Geometry check sheet. Reference: the model listing, model coordinates, mm. Coordinates: 2 decimals unless noted, no trailing zeros. Write each loop counter-clockwise with the first axis right and the second up, starting at its lowest first coordinate (ties: lowest second). Pieces come first, ordered by that corner, then holes. Notation, with made-up numbers: (-4.75, 67.5) -> (10.25, 67.5) arc R19 cw to (10.25, 74.5) -> close; hole circle Ø10 at (45, -1.75). An arc over 180 degrees is marked (long way). Answer in a Markdown table with one row per item. Add a question column.
1. Cross-section at D-D on y = 210. Record the cut outline in (x, z), and give its area (3 significant figures).
2. Depth check by flat-ended pin: P1, Ø1, axis at x = 47, z = 1, coming from the -Y side; P2, Ø2.5, axis at y = 138, z = 2, coming from the +X side; P3, Ø2.5, axis at y = 82.5, z = 2, coming from the +X side; P4, Ø5, axis at x = 31, y = 152, coming from the +Z side. Enter the tip coordinate at first touch or a pass-through.
3. Cross-section at A-A on x = 44. Record the cut outline in (y, z).
4. Cross-section at C-C on y = 27.5. Record the cut outline in (x, z), and give its area (3 significant figures).
5. Scan lines: L1, parallel to X at y = 190, z = 0.75; L2, parallel to Y at x = 45, z = 1.8; L3, parallel to X at y = 135, z = 4.1. Record each from-to range of solid material in increasing order. Write a range as from..to.
6. Cross-section at B-B on z = 3.6. Record the cut outline in (x, y).
```python
from build123d import *

# Parameters (mm, degrees)
BOSS_EXTRU_1_DEPTH = 5


with BuildPart() as part:
    # Esquisse1 → Boss.-Extru.1 (new body)
    with BuildSketch(Plane.XY):
        with BuildLine():
            Line((70.297192809, 66.186397284), (70.297192809, 78.451204868))
            Line((70.297192809, 78.451204868), (39.439293445, 78.451204868))
            Line((39.439293445, 78.451204868), (39.439293445, 90.333987182))
            Line((39.439293445, 90.333987182), (27.572537656, 90.333987182))
            Line((27.572537656, 90.333987182), (27.572537656, 159.717501023))
            Line((27.572537656, 159.717501023), (52.855036633, 185))
            Line((52.855036633, 185), (52.855036633, 260))
            Line((52.855036633, 260), (27.572537656, 260))
            Line((27.572537656, 260), (27.572537656, 270))
            Line((27.572537656, 270), (0, 270))
            Line((0, 270), (0, 0))
            Line((0, 0), (15, 0))
            Line((15, 0), (15, 50))
            ThreePointArc((15, 50), (24.488558001, 59.174106779), (35.670004688, 66.186397284))
            Line((35.670004688, 66.186397284), (70.297192809, 66.186397284))
        make_face()
    extrude(amount=BOSS_EXTRU_1_DEPTH)


solid = part.part
```
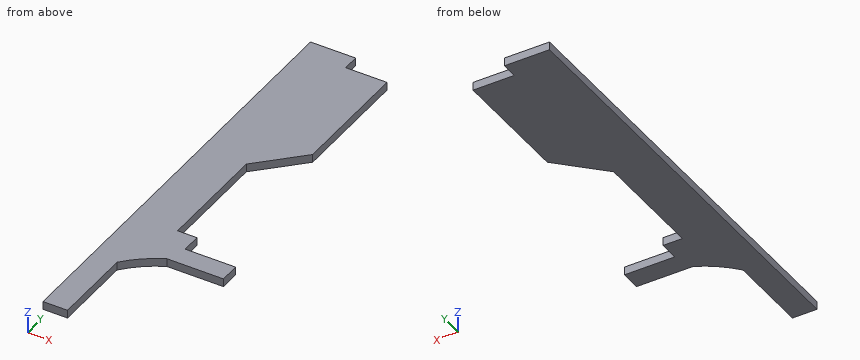
Results found:
| question | item | result |
|---|---|---|
| 1 | outline | (0, 0) -> (52.86, 0) -> (52.86, 5) -> (0, 5) -> close |
| 1 | area | 264 mm^2 |
| 2 | P1 | stops at y = 66.19 |
| 2 | P2 | stops at x = 27.57 |
| 2 | P3 | stops at x = 39.44 |
| 2 | P4 | passes through |
| 3 | outline | (66.19, 0) -> (78.45, 0) -> (78.45, 5) -> (66.19, 5) -> close; (176.14, 0) -> (260, 0) -> (260, 5) -> (176.14, 5) -> close |
| 4 | outline | (0, 0) -> (15, 0) -> (15, 5) -> (0, 5) -> close |
| 4 | area | 75.0 mm^2 |
| 5 | L1 | x = 0..52.86 |
| 5 | L2 | y = 66.19..78.45, 177.14..260 |
| 5 | L3 | x = 0..27.57 |
| 6 | outline | (0, 0) -> (15, 0) -> (15, 50) arc R63.44 cw to (35.67, 66.19) -> (70.3, 66.19) -> (70.3, 78.45) -> (39.44, 78.45) -> (39.44, 90.33) -> (27.57, 90.33) -> (27.57, 159.72) -> (52.86, 185) -> (52.86, 260) -> (27.57, 260) -> (27.57, 270) -> (0, 270) -> close |
